```python
from build123d import *

# Parameters (mm, degrees)
F0_W      = 8.49884
F0_H      = 8.49884
F2_DEPTH  = 3.9624
F3_DEPTH  = 4.2926
F5_DEPTH  = 4.572
F7_DEPTH  = 25.4
F9_DEPTH  = 25.4
F10_W     = 1.016
F10_H     = 2.60096
F11_DEPTH = 4.318


with BuildPart() as f2:
    # F0 (on Front) → F2 (new body)
    with BuildSketch(Plane.XZ):
        Rectangle(F0_W, F0_H)
    extrude(amount=F2_DEPTH)

    # F1 (on face) → F3 (cut)
    with BuildSketch(Plane.XZ):
        Polygon((-4.278509, 4.281422), (-4.251881, 2.683762), (-2.680849, 4.281422), align=None)
    extrude(amount=F3_DEPTH, mode=Mode.SUBTRACT)

    # F4 (on face) → F5 (cut)
    with BuildSketch(Plane.XZ.offset(3.9624)):
        Polygon((4.24942, 4.24942), (2.65176, 4.24942), (4.24942, 2.649474), align=None)
    extrude(amount=-F5_DEPTH, mode=Mode.SUBTRACT)

    # F6 (on face) → F7 (cut)
    with BuildSketch(Plane.XZ.offset(3.9624)):
        Polygon((-4.24942, -2.649474), (-4.24942, -4.24942), (-2.649474, -4.24942), align=None)
    extrude(amount=-F7_DEPTH, mode=Mode.SUBTRACT)

    # F8 (on face) → F9 (cut)
    with BuildSketch(Plane.XZ.offset(3.9624)):
        Polygon((2.667254, -4.24942), (4.24942, -4.24942), (4.24942, -2.667254), align=None)
    extrude(amount=-F9_DEPTH, mode=Mode.SUBTRACT)

    # F10 (on face) → F11 (cut)
    with BuildSketch(Plane.YZ.offset(4.24942)):
        with Locations((-3.631236, 0)):
            Rectangle(F10_W, F10_H)
    extrude(amount=-F11_DEPTH, mode=Mode.SUBTRACT)


solid = f2.part
```
Source: CAD feature listing. Evaluate the final solid. Frame: model axes, mm. A direction names the side the tool comes from. Give positions to 0.01 mm unless a question says otherwise; leave off trailing zeros. Loops run counter-clockwise (first coordinate to the right, second up) from the corner with the lowest first, then second, coordinate; pieces in that order, holes last. Notation, with made-up numbers: (35, 73) - (66, 73) arc R8 cw to (66, 85) - close; hole circle Ø3 at (19.5, 58). An arc over 180 degrees is marked (long way). Use CSV: the item, a comma, the result in double quotes. Start each with the question number.
1. Section B-B (z = -0.75). Output: boundary loops of the cut face in (x, y).
2. Ray query, L1, parallel to Y at x = 1, z = 0; L2, parallel to X at y = -1.8, z = 3; L3, parallel to X at y = -0.25, z = 3.75. Return the intervals inside material, ascending.
3. Section A-A (y = -3.7). Output: boundary loops of the cut face in (x, z).
4. Section C-C (x = 3.25). Output: boundary loops of the cut face in (y, z), then the cut area to 3 significant figures.
5. Reachability of faces 1 (the flat face through (2.1, -3.5, 1.3)), 2 (the flat face through (-4.249, -2, 0)) from +Z, -Z, +X, -X, +Y, -Y: full face, straight path, thin tool, end or side. Return the list, or none.
6. Section D-D (y = -2.8). Output: boundary loops of the cut face in (x, z).
Response:
1,outline,"(-4.25, -3.96) - (-0.07, -3.96) - (-0.07, -3.12) - (4.25, -3.12) - (4.25, 0) - (-4.25, 0) - close"
2,L1,"-3.12 to 0"
2,L2,"-3.94 to 3.9"
2,L3,"-3.2 to 3.15"
3,outline,"(-4.25, -2.65) - (-2.65, -4.25) - (2.67, -4.25) - (4.25, -2.67) - (4.25, -1.3) - (-0.07, -1.3) - (-0.07, 1.3) - (4.25, 1.3) - (4.25, 2.65) - (2.65, 4.25) - (-2.71, 4.25) - (-4.25, 2.69) - close"
4,outline,"(-3.96, -3.67) - (0, -3.67) - (0, 3.65) - (-3.96, 3.65) - (-3.96, 1.3) - (-3.12, 1.3) - (-3.12, -1.3) - (-3.96, -1.3) - close"
4,area,"26.8 mm²"
5,face 1,"+X, -Y"
5,face 2,"+Z, -Z, -X, +Y, -Y"
6,outline,"(-4.25, -2.65) - (-2.65, -4.25) - (2.67, -4.25) - (4.25, -2.67) - (4.25, 2.65) - (2.65, 4.25) - (-2.71, 4.25) - (-4.25, 2.69) - close"
